Verification items for the finished model (mm, model axes). Face numbers are marked on the shaded views. A direction names the side the tool comes from. Give positions to 0.01 mm unless a question says otherwise; leave off trailing zeros. Write each loop counter-clockwise with the first axis right and the second up, starting at its lowest first coordinate (ties: lowest second). Pieces come first, ordered by that corner, then holes. Notation, with made-up numbers: (-26.5, -25) -> (3.5, -25) arc R29 ccw to (3.5, 1) -> close; hole circle Ø4 at (-6, -15.5). An arc over 180 degrees is marked (long way). Answer as CSV lines item,"result".
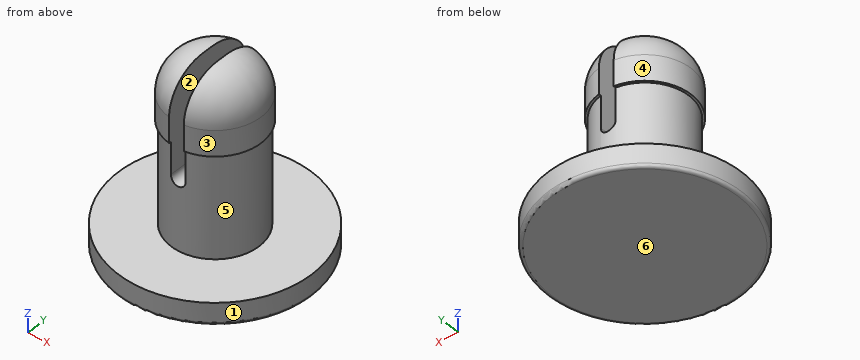
```python
from build123d import *

# Parameters (mm, degrees)
SKETCH2_R               = 7.5
BOSS_EXTRUDE1_DEPTH     = 1.75
FILLET1_R               = 0.25
SKETCH3_R               = 3.405
BOSS_EXTRUDE2_DEPTH     = 8
SKETCH4_R               = 3.575
BOSS_EXTRUDE3_DEPTH     = 5
FILLET3_R               = 3
CUT_EXTRUDE1_DEPTH      = 19.167622299
CUT_EXTRUDE1_DEPTH_BACK = 19.167622299


with BuildPart() as part:
    # Sketch2 → Boss-Extrude1 (new body)
    with BuildSketch(Plane.XY):
        Circle(SKETCH2_R)
    extrude(amount=BOSS_EXTRUDE1_DEPTH)

    # Fillet1
    fillet1_edges = [part.edges().sort_by_distance(p)[0] for p in [
        (-7.5, 0, 0),
    ]]
    fillet(fillet1_edges, radius=FILLET1_R)

    # Sketch3 → Boss-Extrude2 (add)
    with BuildSketch(Plane.XY.offset(1.75)):
        Circle(SKETCH3_R)
    extrude(amount=BOSS_EXTRUDE2_DEPTH)

    # Sketch4 → Boss-Extrude3 (add)
    with BuildSketch(Plane.XY.offset(9.75)):
        Circle(SKETCH4_R)
    extrude(amount=BOSS_EXTRUDE3_DEPTH)

    # Fillet3
    fillet3_edges = [part.edges().sort_by_distance(p)[0] for p in [
        (-3.575, 0, 14.75),
    ]]
    fillet(fillet3_edges, radius=FILLET3_R)

    # Sketch5 → Cut-Extrude1 (cut, two sides: drawn at the far end of the back side and taken through both)
    with BuildSketch(Plane(origin=(0, 0, 0), x_dir=(1, 0, 0), z_dir=(0, 1, 0)).offset(-CUT_EXTRUDE1_DEPTH_BACK)):
        with BuildLine():
            Line((0.575, -14.75), (0.575, -7.25))
            ThreePointArc((0.575, -7.25), (0, -6.675), (-0.575, -7.25))
            Line((-0.575, -7.25), (-0.575, -14.75))
            Line((-0.575, -14.75), (0.575, -14.75))
        make_face()
    extrude(amount=CUT_EXTRUDE1_DEPTH + CUT_EXTRUDE1_DEPTH_BACK, mode=Mode.SUBTRACT)


solid = part.part
```
1) Tool access check on the marked faces 1, 2 and 3. Record the directions out of +Z, -Z, +X, -X, +Y, -Y that give a thin tool (end or side, any length) a straight path to the whole face; none if there is none.
Reported:
face 1,"+Z, -Z"
face 2,"+Z, +Y, -Y"
face 3,"+Z, +X"
2) Section check C-C (z = 1.5). Record the boundary of the cut face in (x, y), and give its area (3 significant figures).
Reported:
outline,"circle Ø15 at (0, 0)"
area,"177 mm²"
3) Section check A-A (x = 0). Record the boundary of the cut face in (y, z) (3 decimals), and give its area (3 significant figures).
Reported:
outline,"(-7.5, 0.25) arc R0.25 ccw to (-7.25, 0) -> (7.25, 0) arc R0.25 ccw to (7.5, 0.25) -> (7.5, 1.75) -> (3.405, 1.75) -> (3.405, 6.675) -> (-3.405, 6.675) -> (-3.405, 1.75) -> (-7.5, 1.75) -> close"
area,"59.8 mm²"
4) Scan lines: line 1 along Z through (x, y) = (6.25, 2.5); line 2 along X through (y, z) = (3, 11.25) (3 decimals); line 3 along X through (y, z) = (0.25, 1.5). Record each from-to range of solid material in increasing order.
Reported:
line 1,"0 to 1.75"
line 2,"-1.944 to -0.575, 0.575 to 1.944"
line 3,"-7.5 to 7.5"
5) Draft check along Z on the marked faces 4, 5 and 6. Enter one of: +Z half, -Z half, draft (parallel to the pull), parting line (faces both ways), or undercut.
Reported:
face 4,"draft"
face 5,"undercut"
face 6,"-Z half"
6) Section check B-B (z = 8). Record the boundary of the cut face in (x, y) (3 decimals).
Reported:
outline,"(-0.575, -3.356) -> (-0.575, 3.356) arc R3.405 ccw to start; (0.575, -3.356) arc R3.405 ccw to (0.575, 3.356) -> close"
7) Depth check by flat-ended pin: pin 1 (1 mm diameter, centred on x = -2, y = -2.5, fed in from +Z); pin 2 (8 mm diameter, centred on y = 1, z = 12, fed in from +X) (3 decimals); pin 3 (4 mm diameter, centred on x = -1, z = 10, fed in from -Y). Enter the tip coordinate at first touch or a pass-through.
Reported:
pin 1,"z = 13.87"
pin 2,"x = 3.575"
pin 3,"y = -3.53"
